Autodesk Inventor part; units mm, degrees
ref_plane "YZ Plane" through (0, 0, 0) normal (1, 0, 0) x (0, 1, 0)
ref_plane "XZ Plane" through (0, 0, 0) normal (0, 1, 0) x (-1, 0, 0)
ref_plane "XY Plane" through (0, 0, 0) normal (0, 0, 1) x (1, 0, 0)
sketch "Sketch1" plane through (0, 0, 0) normal (0, 1, 0) x (-1, 0, 0)
  line L0 (0, 0) -> (25, 0)
  line L1 (25, 0) -> (25, -25)
  line L2 (25, -25) -> (0, -25)
  line L3 (0, -25) -> (0, 0)
  line L4 (22, -22) -> (22, -3)
  line L5 (22, -3) -> (3, -3)
  line L6 (3, -3) -> (3, -22)
  line L7 (3, -22) -> (22, -22)
  dimension "d0" = 25
  dimension "d1" = 25
  dimension "d2" = 3
extrude "Extrusion1" add sketch "Sketch1" along normal blind 80
sketch "Sketch2" plane through (0, 0, 0) normal (1, 0, 0) x (0, 0, -1)
  line L0 (0, 0) -> (25, 0)
  line L1 (25, 0) -> (25, 80)
  line L2 (0, 80) -> (25, 80)
  line L3 (0, 0) -> (0, 80)
  line L4 (0, 0) -> (0, 80)
  line L5 (0, 80) -> (25, 55)
  line L6 (0, 80) -> (35.3553, 80) construction
  dimension "d5" = 45
extrude "Extrusion2" cut sketch "Sketch2" against normal blind 80 contours L2 L1 L5
properties part number "P403" material "Aluminum 6061"
Work out the finished part from the listing and answer in its coordinate system (mm). A direction names the side the tool comes from. Give positions to 0.01 mm unless a question says otherwise; leave off trailing zeros. Loops run counter-clockwise (first coordinate to the right, second up) from the corner with the lowest first, then second, coordinate; pieces in that order, holes last. Notation, with made-up numbers: (-10.75, -25) -> (17.25, -25) arc R22 ccw to (17.25, -10) -> close; hole circle Ø3 at (10, 73). An arc over 180 degrees is marked (long way). Use a Markdown table: item, result. Add a question column.
1) The part is cut by section B-B, the plane y = 9.5. Determine the outline of the cut face in (x, z), plus the area to 3 significant figures.
2) The part is cut by section C-C, the plane x = -14. Determine the outline of the cut face in (y, z).
3) The part is cut by section D-D, the plane y = 63. Determine the outline of the cut face in (x, z), plus the area to 3 significant figures.
4) Each of these flat-tipped pins is pushed along its axis until it touches: P1, Ø1, axis at x = -20.5, z = -15.5, coming from the -Y side; P2, Ø1, axis at x = -2.5, z = -3, coming from the +Y side. Where does it stop, or does it pass through?
5) For a pull along Z with two mould halves and no side action, classify faces 3 (the flat face through (-22, 29, -13)), 4 (the flat face through (-23, 68, -12)), 5 (the flat face through (0, 31, -13)) as +Z half, -Z half, draft (parallel to the pull), parting line (faces both ways), or undercut.
6) The part is cut by section A-A, the plane z = -7.25. Determine the outline of the cut face in (x, y).
7) Consider line 1 along X through (y, z) = (39.5, -16.75); line 2 along Z through (x, y) = (-14.25, 64.5). Determine where each line is inside the solid, lowest interval first.
8) Which of the six approach directions +Z, -Z, +X, -X, +Y, -Y give full straight-line access (tool end or side, diameter ignored) to faces 1 (the flat face through (-3, 29, -12)), 2 (the flat face through (-23, 0, -12))?
Reported:
| question | item | result |
|---|---|---|
| 1 | outline | (-25, -25) -> (0, -25) -> (0, 0) -> (-25, 0) -> close; hole (-22, -22) -> (-3, -22) -> (-3, -3) -> (-22, -3) -> close |
| 1 | area | 264 mm^2 |
| 2 | outline | (0, -25) -> (55, -25) -> (58, -22) -> (0, -22) -> close; (0, -3) -> (77, -3) -> (80, 0) -> (0, 0) -> close |
| 3 | outline | (-25, -17) -> (-22, -17) -> (-22, -3) -> (-3, -3) -> (-3, -17) -> (0, -17) -> (0, 0) -> (-25, 0) -> close |
| 3 | area | 159 mm^2 |
| 4 | P1 | passes through |
| 4 | P2 | stops at y = 77.5 |
| 5 | face 3 | undercut |
| 5 | face 4 | -Z half |
| 5 | face 5 | draft |
| 6 | outline | (-25, 0) -> (-22, 0) -> (-22, 72.75) -> (-25, 72.75) -> close; (-3, 0) -> (0, 0) -> (0, 72.75) -> (-3, 72.75) -> close |
| 7 | line 1 | x = -25 to -22, -3 to 0 |
| 7 | line 2 | z = -3 to 0 |
| 8 | face 1 | +Y, -Y |
| 8 | face 2 | +Z, -Z, +X, -X, -Y |
